CAD build for the part. Positions are in the model's coordinates, mm. Give positions to 0.01 mm unless a question says otherwise; leave off trailing zeros. Write each loop counter-clockwise with the first axis right and the second up, starting at its lowest first coordinate (ties: lowest second). Pieces come first, ordered by that corner, then holes. Notation, with made-up numbers: (-4.75, -21.75) - (32.25, -21.75) arc R10 ccw to (32.25, -5.75) - close; hole circle Ø7 at (22, 25.5). An arc over 180 degrees is marked (long way). Answer as a JSON object with one key per item and string values.
from build123d import *

# Parameters (mm, degrees)
SALIENTE_EXTRUIR1_DEPTH = 276.5
REDONDEO1_R             = 0.5
REDONDEO2_R             = 1
REDONDEO3_R             = 1.5
REDONDEO4_R             = 1.5


with BuildPart() as part:
    # Croquis1 → Saliente-Extruir1 (new body)
    with BuildSketch(Plane(origin=(0, 0, 0), x_dir=(1, 0, 0), z_dir=(0, 1, 0))):
        Polygon((0, 0), (0, 31.5), (-10.4, 31.5), (-10.4, 30), (-1.5, 30), (-1.5, 18.5), (-3.8, 18.5), (-3.8, 19.3), (-4.7, 19.3), (-4.7, 17.5), (-1.5, 17.5), (-1.5, 12.5), (-4.7, 12.5), (-4.7, 10.7), (-3.8, 10.7), (-3.8, 11.5), (-1.5, 11.5), (-1.5, 0), align=None)
    extrude(amount=SALIENTE_EXTRUIR1_DEPTH)

    # Redondeo1
    redondeo1_edges = [part.edges().sort_by_distance(p)[0] for p in [
        (-4.7, 138.25, -10.7),
        (-4.7, 138.25, -19.3),
    ]]
    fillet(redondeo1_edges, radius=REDONDEO1_R)

    # Redondeo2
    redondeo2_edges = [part.edges().sort_by_distance(p)[0] for p in [
        (-1.5, 138.25, -12.5),
        (-1.5, 138.25, -17.5),
    ]]
    fillet(redondeo2_edges, radius=REDONDEO2_R)

    # Redondeo3
    redondeo3_edges = [part.edges().sort_by_distance(p)[0] for p in [
        (-1.5, 138.25, -30),
    ]]
    fillet(redondeo3_edges, radius=REDONDEO3_R)

    # Redondeo4
    redondeo4_edges = [part.edges().sort_by_distance(p)[0] for p in [
        (0, 138.25, -31.5),
    ]]
    fillet(redondeo4_edges, radius=REDONDEO4_R)


solid = part.part
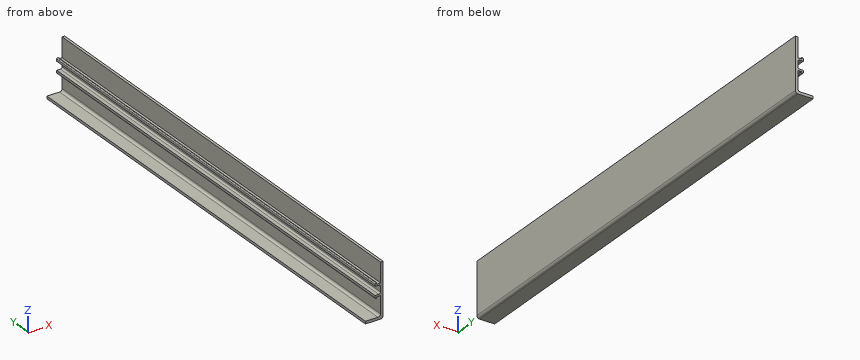
(1) Probe L1, parallel to Z at x = -3.5, y = 92.5; L2, parallel to Z at x = -4, y = 100; L3, parallel to X at y = 174.5, z = -7. List the from-to ranges inside material, lowest first. Write a range as [from, to].
Answer key:
{"L1": "z = [-31.5, -30], [-18.5, -17.5], [-12.5, -11.5]", "L2": "z = [-31.5, -30], [-19.3, -17.5], [-12.5, -10.7]", "L3": "x = [-1.5, 0]"}
(2) Flat gauge pins, fed straight in: P1, Ø0.7, axis at y = 92.5, z = -18, coming from the -X side; P2, Ø6, axis at x = -5, y = 78, coming from the +Z side; P3, Ø6, axis at x = -5.5, z = -26, coming from the +Y side; P4, Ø0.9, axis at y = 192, z = -14.5, coming from the -X side. Where does each tip first touch, or does it go through?
Answer key:
{"P1": "stops at x = -4.7", "P2": "stops at z = -10.7", "P3": "passes through", "P4": "stops at x = -1.5"}
(3) Saw through at A-A, the plane y = 90. Give the cut face in (x, z).
Answer key:
{"outline": "(-10.4, -31.5) - (-1.5, -31.5) arc R1.5 ccw to (0, -30) - (0, 0) - (-1.5, 0) - (-1.5, -11.5) - (-3.8, -11.5) - (-3.8, -10.7) - (-4.2, -10.7) arc R0.5 ccw to (-4.7, -11.2) - (-4.7, -12.5) - (-2.5, -12.5) arc R1 cw to (-1.5, -13.5) - (-1.5, -16.5) arc R1 cw to (-2.5, -17.5) - (-4.7, -17.5) - (-4.7, -18.8) arc R0.5 ccw to (-4.2, -19.3) - (-3.8, -19.3) - (-3.8, -18.5) - (-1.5, -18.5) - (-1.5, -28.5) arc R1.5 cw to (-3, -30) - (-10.4, -30) - close"}
(4) Saw through at C-C, the plane x = -8.75. Give the cut face in (y, z), and give its area (3 significant figures).
Answer key:
{"outline": "(0, -31.5) - (276.5, -31.5) - (276.5, -30) - (0, -30) - close", "area": "415 mm²"}
(5) Saw through at B-B, the plane z = -5. Give the cut face in (x, y).
Answer key:
{"outline": "(-1.5, 0) - (0, 0) - (0, 276.5) - (-1.5, 276.5) - close"}
